```python
from build123d import *

# Parameters (mm, degrees)
SKETCH4_R          = 1.36
CUT_EXTRUDE1_DEPTH = 4
SKETCH5_R          = 1.36
CUT_EXTRUDE2_DEPTH = 4
SKETCH6_W          = 5.726444475
SKETCH6_H          = 2.29057779
CUT_EXTRUDE3_DEPTH = 3.5
FILLET1_R          = 1


with BuildPart() as part:
    # Sketch1 → Revolve1 (revolve)
    with BuildSketch(Plane(origin=(0, 0, 0), x_dir=(0, 0, -1), z_dir=(1, 0, 0))):
        Polygon((15.9, 0), (3.25, 0), (3.25, -0.75), (3.5, -0.75), (3.5, -1.2), (3.2, -1.5), (2.55, -1.5), (2.55, 14.175), (2.775, 14.4), (3.275, 14.4), (3.5, 14.175), (3.5, 14.805662433), (3.75, 14.95), (14.5, 14.95), (17.35, 13.2), (17.35, 11.2), (17.415, 11.2), (17.415, 5.45), (16.415, 5.45), (16.415, 11.42717663), (12.5, 13.831123999), (12.5, 4.95), (12.5, 2), (15.9, 2), (15.9, 4.95), (17.415, 4.95), (17.415, 1.515), align=None)
    revolve(axis=Axis((0, 0, 0), (0, 1, 0)))

    # Sketch3 → Cut-Revolve1 (revolve, cut)
    with BuildSketch(Plane(origin=(0, 0, 0), x_dir=(0, 0, -1), z_dir=(1, 0, 0))):
        Polygon((5.5, 0), (5.5, -0.625659235), (3.25, -0.071654916), (3.25, 0.040355339), (3.285355339, 0.005), (3.714644661, 0.005), (3.75, 0.040355339), (3.75, 0.065), (5, 0.065), (5, 0.040355339), (5.035355339, 0.005), (5.464644661, 0.005), (5.5, 0.040355339), align=None)
    revolve(axis=Axis((0, 0, 0), (0, 1, 0)), mode=Mode.SUBTRACT)

    # Sketch4 → Cut-Extrude1 (cut)
    with BuildSketch(Plane(origin=(0, 14.95, 0), x_dir=(1, 0, 0), z_dir=(0, 1, 0))):
        with Locations((0, 8)):
            Circle(SKETCH4_R)
        with Locations((8, 0)):
            Circle(SKETCH4_R)
        with Locations((0, -8)):
            Circle(SKETCH4_R)
        with Locations((-8, 0)):
            Circle(SKETCH4_R)
    extrude(amount=-CUT_EXTRUDE1_DEPTH, mode=Mode.SUBTRACT)

    # Sketch5 → Cut-Extrude2 (cut)
    with BuildSketch(Plane.XZ):
        with Locations((-6.717514421, -6.717514421)):
            Circle(SKETCH5_R)
        with Locations((5.656854249, -5.656854249)):
            Circle(SKETCH5_R)
        with Locations((-5.656854249, 5.656854249)):
            Circle(SKETCH5_R)
        with Locations((6.717514421, 6.717514421)):
            Circle(SKETCH5_R)
    extrude(amount=-CUT_EXTRUDE2_DEPTH, mode=Mode.SUBTRACT)

    # Sketch6 → Cut-Extrude3 (cut, symmetric)
    with BuildSketch(Plane(origin=(0, 0, 0), x_dir=(0, 0, -1), z_dir=(1, 0, 0))):
        with Locations((-15.363222238, 4.025390462)):
            Rectangle(SKETCH6_W, SKETCH6_H)
    extrude(amount=CUT_EXTRUDE3_DEPTH, both=True, mode=Mode.SUBTRACT)

    # Fillet1
    fillet1_edges = [part.edges().sort_by_distance(p)[0] for p in [
        (-3.5, 2.880101567, 16.284831695),
        (3.5, 2.880101567, 16.284831695),
    ]]
    fillet(fillet1_edges, radius=FILLET1_R)


solid = part.part
```
Geometry check sheet. Reference: the model listing, model coordinates, mm. A direction names the side the tool comes from. Round coordinates to 2 decimals unless told otherwise and drop trailing zeros. Order: outer loops, then holes, each group sorted by start corner. A loop starts at its lowest first (then second) coordinate and runs counter-clockwise, first axis right, second up. Notation, with made-up numbers: (-26.5, -27) - (-2.5, -27) arc R25 ccw to (-2.5, -3) - close; hole circle Ø7 at (-6, -20.75). An arc over 180 degrees is marked (long way). Use a Markdown table: item, result. Add a question column.
(1) Release check for a two-part mould opening along X. For faces 1 (the cylindrical face through (1.341, -0.978, -3.233)), 2 (the flat face through (0, 0, -7)), 3 (the cylindrical face through (-4.776, 3.496, -15.166)) record: pulls with the +X half, pulls with the -X half, needs draft (parallel to the pull), parting line crosses it, or undercut.
(2) Sectioned sample at A-A, the plane y = 0.75. Enter the section's corners in (x, z).
(3) Depth check by flat-ended pin: pin 1 (3 mm diameter, centred on x = -5.5, z = 6, fed in from -Y); pin 2 (1.4 mm diameter, centred on x = 7, z = 6.5, fed in from -Y); pin 3 (0.5 mm diameter, centred on x = -1, z = 16.5, fed in from +Y); pin 4 (2 mm diameter, centred on x = 0, z = -1, fed in from -Y). Enter the tip coordinate at first touch or a pass-through.
(4) Material ranges on line 1 along Y through (x, z) = (-13.5, -0.5); line 2 along X through (y, z) = (6.75, 11); line 3 along X through (y, z) = (9.75, 4), recorded low to high. Write a range as [from, to].
(5) Tool access check on faces 4 (the cylindrical face through (-5.23, 3.21, -16.61)), 5 (the cylindrical face through (-3.755, 7.998, -11.923)), 6 (the flat face through (-4, 0.065, 1)), 7 (the cylindrical face through (-3.199, 3.165, 16.36)), 8 (the cylindrical face through (9.256, 12.978, 0.521)). Record the directions out of +Z, -Z, +X, -X, +Y, -Y that give a thin tool (end or side, any length) a straight path to the whole face; none if there is none.
Answers below:
| question | item | result |
|---|---|---|
| 1 | face 1 | parting line crosses it |
| 1 | face 2 | needs draft |
| 1 | face 3 | undercut |
| 2 | outline | circle Ø33.3 at (0, 0); hole circle Ø2.72 at (-6.72, -6.72); hole circle Ø2.72 at (-5.66, 5.66); hole circle Ø5.1 at (0, 0); hole circle Ø2.72 at (5.66, -5.66); hole circle Ø2.72 at (6.72, 6.72) |
| 3 | pin 1 | y = 0 |
| 3 | pin 2 | y = 4 |
| 3 | pin 3 | y = 13.86 |
| 3 | pin 4 | through |
| 4 | line 1 | [0, 2], [13.21, 14.95] |
| 4 | line 2 | [-13.5, -12.18], [-5.94, 5.94], [12.18, 13.5] |
| 4 | line 3 | [-16.95, -15.92], [-11.84, 11.84], [15.92, 16.95] |
| 5 | face 4 | +Y, -Y |
| 5 | face 5 | none |
| 5 | face 6 | -Y |
| 5 | face 7 | +Z |
| 5 | face 8 | +Y |
